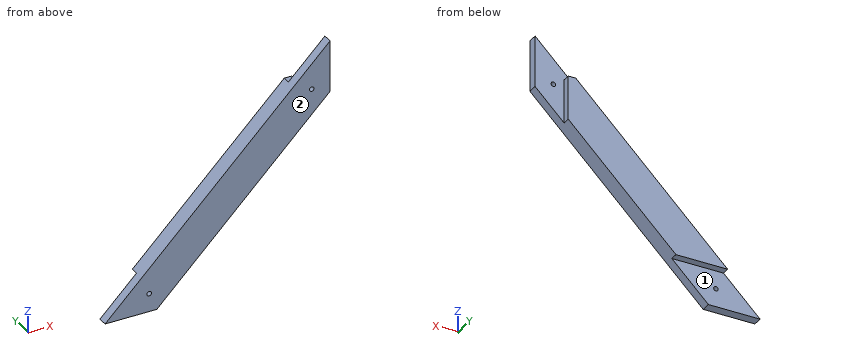
```python
from build123d import *

# Parameters (mm, degrees)
F1_DEPTH = 22.5
F3_DEPTH = 20
F5_DEPTH = 20
F6_R     = 6
F7_DEPTH = 25
F8_R     = 6
F9_DEPTH = 25


with BuildPart() as f1:
    # F0 (on Front) → F1 (new body, symmetric)
    with BuildSketch(Plane.XZ):
        Polygon((264.205321, 195.615963), (264.205321, 332.794679), (-332.794679, -264.205321), (-195.615963, -264.205321), align=None)
    extrude(amount=F1_DEPTH, both=True)

    # F2 (on face) → F3 (cut)
    with BuildSketch(Plane(origin=(0, 22.5, 0), x_dir=(-1, 0, 0), z_dir=(0, 1, 0))):
        Polygon((-187.205321, 235.794679), (-167.205321, 235.794679), (-264.205321, 332.794679), (-264.205321, 195.615963), (-187.205321, 118.615963), align=None)
    extrude(amount=-F3_DEPTH, mode=Mode.SUBTRACT)

    # F4 (on face) → F5 (cut)
    with BuildSketch(Plane(origin=(0, 22.5, 0), x_dir=(-1, 0, 0), z_dir=(0, 1, 0))):
        Polygon((332.794679, -264.205321), (235.794679, -167.205321), (98.615963, -167.205321), (195.615963, -264.205321), align=None)
    extrude(amount=-F5_DEPTH, mode=Mode.SUBTRACT)

    # F6 (on face) → F7 (cut, through all)
    with BuildSketch(Plane(origin=(0, 2.5, 0), x_dir=(-1, 0, 0), z_dir=(0, 1, 0))):
        with Locations((-215.705321, 215.705321)):
            Circle(F6_R)
    extrude(amount=-F7_DEPTH, mode=Mode.SUBTRACT)

    # F8 (on face) → F9 (cut, through all)
    with BuildSketch(Plane(origin=(0, 2.5, 0), x_dir=(-1, 0, 0), z_dir=(0, 1, 0))):
        with Locations((215.705321, -215.705321)):
            Circle(F8_R)
    extrude(amount=-F9_DEPTH, mode=Mode.SUBTRACT)


solid = f1.part
```
Geometry: final body of the model. Coordinates: model frame, mm. Face numbers are marked on the shaded views. A direction names the side the tool comes from. Round coordinates to 2 decimals unless told otherwise and drop trailing zeros. Order: outer loops, then holes, each group sorted by start corner. A loop starts at its lowest first (then second) coordinate and runs counter-clockwise, first axis right, second up. Notation, with made-up numbers: (-26, 49.5) -> (2, 49.5) arc R32 cw to (2, 82.5) -> close; hole circle Ø9 at (45.5, -32). An arc over 180 degrees is marked (long way). Use CSV: the item, a comma, the result in double quotes. Start each with the question number.
1) Set-up query: the marked faces 1 and 2. Return all of +Z, -Z, +X, -X, +Y, -Y with unobstructed straight access to the full face (end or side cutting, diameter ignored); none if empty.
2) Section C-C (z = 46). Return the cut outline in (x, y), and give its area (3 significant figures).
3) Section B-B (x = -184). Return the cut outline in (y, z), and give its area (3 significant figures).
4) Section A-A (y = 15). Return the cut outline in (x, z), and give its area (3 significant figures).
5) First-contact query: pin 1 Ø1.5 at (y, z) = (9.5, 207) entering from +X; pin 2 Ø5 at (x, y) = (166, 5) entering from +Z; pin 3 Ø15.5 at (x, z) = (215.71, 215.71) entering from +Y. Flat tips, straight axial feed; report the tip coordinate or a pass-through.
6) Material intervals for line 1 along X through (y, z) = (-13, 217); line 2 along Y through (x, z) = (227.5, 202.5); line 3 along Z through (x, y) = (-159, 9.5), sorted ascending. Write a range as from..to.
7) Section D-D (x = 23). Return the cut outline in (y, z), and give its area (3 significant figures).
Returned:
1,face 1,"-Z, +X, -X, +Y"
1,face 2,"+Z, -Z, +X, -X, -Y"
2,outline,"(-22.59, -22.5) -> (114.59, -22.5) -> (114.59, 22.5) -> (-22.59, 22.5) -> close"
2,area,"6,170 mm²"
3,outline,"(-22.5, -252.59) -> (2.5, -252.59) -> (2.5, -167.21) -> (22.5, -167.21) -> (22.5, -115.41) -> (-22.5, -115.41) -> close"
3,area,"4,470 mm²"
4,outline,"(-235.79, -167.21) -> (-98.62, -167.21) -> (187.21, 118.62) -> (187.21, 235.79) -> (167.21, 235.79) -> close"
4,area,"48,400 mm²"
5,pin 1,"stops at x = 187.21"
5,pin 2,"stops at z = 235.79"
5,pin 3,"stops at y = 2.5"
6,line 1,"x = 148.41..209.85, 221.56..264.21"
6,line 2,"y = -22.5..2.5"
6,line 3,"z = -167.21..-90.41"
7,outline,"(-22.5, -45.59) -> (22.5, -45.59) -> (22.5, 91.59) -> (-22.5, 91.59) -> close"
7,area,"6,170 mm²"
